Could you check a few things on this model? Use its own coordinates, in mm. Give positions to 0.01 mm unless a question says otherwise; leave off trailing zeros. Loops run counter-clockwise (first coordinate to the right, second up) from the corner with the lowest first, then second, coordinate; pieces in that order, holes last. Notation, with made-up numbers: (8.25, -11.75) -> (41.25, -11.75) arc R6 cw to (41.25, -0.75) -> close; hole circle Ø7 at (-26.5, 85). An arc over 180 degrees is marked (long way). Write item = value, one per line. Start each with the question number.
1) I want a section at C-C (z = 1.05). Count the separate pieces of the cut face and the enclosed holes in it, and give its area (3 significant figures).
2) I want a section at A-A (x = 160). List the corners of the cut face in (y, z) for me (3 decimals).
3) I'm going to push flat-ended pins straight in: pin 1 Ø1.5 at (x, y) = (117, 105) entering from -Z; pin 2 Ø1.6 at (y, z) = (13.5, 2) entering from +X; pin 3 Ø3 at (x, y) = (152.4, 106.807) entering from -Z. Where does each tip first touch, or does it pass through?
4) I need wall thicknesses on probe 1 along Y at (x, z) = (190.5, 2.55) (3 decimals); probe 2 along Y at (x, z) = (107.95, 1.85); probe 3 along X at (y, z) = (12.5, 2.7). Which ranges of each line are inside material? Lowest first, please. Write a range as from..to.
5) I want a section at B-B (y = 26). List the corners of the cut face in (x, z) for me (3 decimals).
6) If we mould it in two halves opening along Y, with no side actions, what happens to faces 1 (the face through (24.32, 56.86, 1.57)), 2 (the face through (36.573, 34.472, 1.61)), 3 (the face through (106, 82, 3.175))? For each: +Y half, -Y half, draft (parallel to the pull), parting line (faces both ways), or undercut.
Autodesk Inventor part; units mm, degrees
ref_plane "YZ Plane" through (0, 0, 0) normal (1, 0, 0) x (0, 1, 0)
ref_plane "XZ Plane" through (0, 0, 0) normal (0, 1, 0) x (-1, 0, 0)
ref_plane "XY Plane" through (0, 0, 0) normal (0, 0, 1) x (1, 0, 0)
sketch "Sketch1" plane through (0, 0, 0) normal (0, 0, 1) x (1, 0, 0)
  line L0 (0, 0) -> (215.9, 0)
  line L1 (215.9, 0) -> (215.9, 152.4)
  line L2 (215.9, 152.4) -> (0, 152.4)
  line L3 (0, 152.4) -> (0, 0)
  dimension "d0" = 215.9
  dimension "d1" = 152.4
extrude "Extrusion1" add sketch "Sketch1" along normal blind 3.175
sketch "Sketch2" plane through (0, 0, 3.175) normal (0, 0, 1) x (1, 0, 0)
  line L0 (215.9, 152.4) -> (0, 152.4) construction
  line L1 (107.95, 152.4) -> (107.95, 0) construction
  line L2 (0, 0) -> (215.9, 0)
  point P0 (25.273, 59.8875)
  point P1 (77.3049, 7.5)
  point P2 (190.627, 59.8875)
  point P3 (138.5951, 7.5)
  dimension "d5" = 30.6451
  dimension "d7" = 82.677
  dimension "d9" = 52.3875
  dimension "d10" = 7.5
hole "Hole1" at (25.273, 59.8875, 3.175) at (77.3049, 7.5, 3.175) at (190.627, 59.8875, 3.175) at (138.5951, 7.5, 3.175) direction (0, 0, -1) diameter 6.35 end through all
sketch "Sketch3" plane through (0, 0, 3.175) normal (0, 0, 1) x (1, 0, 0)
  line L0 (215.9, 152.4) -> (0, 152.4)
  line L1 (107.95, 152.4) -> (107.95, 0)
  line L2 (0, 0) -> (215.9, 0)
  line L3 (21.4376, 59.8875) -> (76.2, 7.5) construction
  line L4 (0, 152.4) -> (0, 0)
  line L5 (0, 130.175) -> (0, 78.2462)
  line L6 (3.175, 133.35) -> (107.95, 133.35)
  line L7 (0, 133.35) -> (0, 125.3708)
  line L8 (194.4624, 59.8875) -> (139.7, 7.5) construction
  line L9 (215.9, 152.4) -> (215.9, 78.2462)
  line L10 (215.9, 133.35) -> (215.9, 76.9596)
  line L11 (212.725, 133.35) -> (107.95, 133.35)
  line L12 (215.9, 130.175) -> (215.9, 125.3708)
  line L13 (75.9713, 0) -> (107.95, 0)
  line L14 (139.9287, 0) -> (107.95, 0)
  line L15 (215.9, 0) -> (215.9, 152.4)
  line L16 (107.95, 56.0437) -> (190.627, 56.0437) construction
  line L17 (0, 0) -> (215.9, 0)
  line L18 (143.7779, 0) -> (215.9, 69.9366)
  line L19 (72.1221, 0) -> (0, 69.9366)
  line L20 (0, 152.4) -> (0, 0)
  line L21 (72.1221, 0) -> (107.95, 0)
  line L22 (3.175, 133.35) -> (0, 133.35)
  line L23 (212.725, 133.35) -> (215.9, 133.35)
  point P0 (74.6275, 0)
  point P1 (0, 76.9596)
  point P2 (77.9849, 0)
  dimension "d20" = 19.05
  dimension "d36" = 135.881
  dimension "d37" = 135.881
  dimension "d41" = 35.8279
sketch "Sketch4" plane through (0, 0, 3.175) normal (0, 0, 1) x (1, 0, 0)
  arc A0 (80.4798, 20.1806) -> (74.13, 20.1806) centre (77.3049, 20.2) ccw
  circle A1 centre (77.3049, 7.5) radius 3.175
  circle A2 centre (77.3049, 7.5) radius 3.175
  line L0 (3.175, 133.35) -> (212.725, 133.35)
  line L1 (107.95, 133.35) -> (107.95, 0) construction
  line L2 (0, 0) -> (215.9, 0)
  arc A3 (141.77, 20.176) -> (135.4202, 20.176) centre (138.5951, 20.2) ccw
  arc A4 (74.1357, 7.5165) -> (80.474, 7.4806) centre (77.3049, 7.5) ccw
  circle A5 centre (138.5951, 7.5) radius 3.175
  arc A6 (135.4202, 7.5433) -> (141.77, 7.5433) centre (138.5951, 7.5) ccw
  line L3 (141.77, 20.176) -> (141.77, 7.476)
  circle A7 centre (138.5951, 7.5) radius 3.175
  line L4 (141.77, 20.176) -> (154.47, 20.176) construction
  line L5 (135.4202, 20.176) -> (135.4202, 7.476)
  line L6 (135.4202, 20.176) -> (148.1202, 20.176) construction
  line L7 (80.4798, 20.1806) -> (80.4798, 7.4806)
  line L8 (80.4798, 20.1806) -> (93.1798, 20.1806) construction
  line L9 (74.13, 20.1806) -> (74.1358, 7.4806)
  line L10 (74.13, 20.1806) -> (86.83, 20.1806) construction
  line L11 (74.13, 20.1806) -> (80.4798, 20.1806)
  line L12 (74.1358, 7.4806) -> (80.4798, 7.4806)
  line L13 (135.4202, 7.476) -> (141.77, 7.476)
  line L14 (135.4202, 20.176) -> (141.77, 20.176)
  line L15 (107.95, 0) -> (107.95, 152.4)
  line L16 (215.9, 152.4) -> (0, 152.4)
  line L17 (138.5951, 7.5) -> (107.95, 7.5)
  line L18 (138.5951, 20.2) -> (107.95, 20.2)
  line L19 (138.5951, 20.2) -> (169.2402, 20.2) construction
  point P0 (75.9713, 0)
  point P1 (139.9287, 0)
  point P2 (136.525, 7.4971)
  dimension "d29" = 6.35
  dimension "d30" = 12.7
  dimension "d44" = 90
  dimension "d45" = 90
  dimension "d46" = 90
  dimension "d48" = 12.7
  dimension "d49" = 12.7
  dimension "d50" = 12.7
  dimension "d117" = 180
extrude "Extrusion3" cut sketch "Sketch3" against normal blind 25.4 contours L9 L23 L11 L1 L0 | L1 L6 L22 L4 L0 | L2 L4 L19 | L18 L15 L2
extrude "Extrusion5" cut sketch "Sketch4" against normal blind 25.4 contours L11 A0 | L7 A1 L9 L11 | A1 L12 A4 L9 | L9 A4 L12 A1 | A4 L12 | L14 A3 | L3 A5 L5 L14 | A5 L13 | A5 L13
fillet "Fillet1" radius 3.175 6 edges at (0, 69.9366, 1.5875) (0, 133.35, 1.5875) (215.9, 133.35, 1.5875) (215.9, 69.9366, 1.5875) (143.7779, 0, 1.5875) (72.1221, 0, 1.5875)
sketch "Sketch5" plane through (0, 0, 3.175) normal (0, 0, 1) x (1, 0, 0)
  line L0 (73.4087, 0) -> (142.4913, 0)
  line L1 (73.4087, 0) -> (142.4913, 0)
  line L2 (107.95, 0) -> (107.95, 133.35)
  line L3 (212.725, 133.35) -> (3.175, 133.35)
  line L4 (107.95, 0) -> (241.3, 0) construction
  line L5 (107.95, 0) -> (107.95, 30.691)
  line L6 (122.6947, 0) -> (122.6947, 60.5028)
  line L7 (122.6947, 0) -> (183.1975, 0) construction
  circle A0 centre (107.95, 15.3455) radius 1.4986
  point P0 (0, 0)
  point P1 (93.2053, 60.5028)
  dimension "d56" = 90
  dimension "d58" = 90
  dimension "d59" = 60.5028
  dimension "d60" = 2.9972
  dimension "d61" = 14.7447
  dimension "d62" = 14.7447
  dimension "d63" = 60.5028
hole "Hole2" at (107.95, 15.3455, 3.175) at (93.2053, 60.5028, 3.175) at (122.6947, 60.5028, 3.175) at (107.95, 15.3455, 3.175) at (122.6947, 60.5028, 3.175) direction (0, 0, -1) diameter 2.9972 end through all
sketch "Sketch7" plane through (0, 0, 3.175) normal (0, 0, 1) x (1, 0, 0)
  line L0 (212.725, 133.35) -> (3.175, 133.35)
  line L1 (0, 130.175) -> (0, 71.2804)
  point P0 (0, 0)
  point P1 (19.05, 126.1872)
  point P2 (38.1, 106.807)
  point P3 (57.15, 126.1872)
  point P4 (76.2, 106.807)
  point P5 (95.25, 126.1872)
  point P6 (114.3, 106.807)
  point P7 (133.35, 126.1872)
  point P8 (152.4, 106.807)
  point P9 (171.45, 126.1872)
  point P10 (190.5, 106.807)
  dimension "d83" = 7.1628
  dimension "d84" = 19.05
  dimension "d85" = 7.1628
  dimension "d89" = 26.543
  dimension "d90" = 26.543
  dimension "d94" = 38.1
  dimension "d95" = 57.15
  dimension "d96" = 76.2
  dimension "d97" = 7.1628
  dimension "d98" = 95.25
  dimension "d99" = 26.543
  dimension "d100" = 114.3
  dimension "d102" = 7.1628
  dimension "d103" = 133.35
  dimension "d104" = 26.543
  dimension "d105" = 152.4
  dimension "d106" = 7.1628
  dimension "d107" = 171.45
  dimension "d108" = 26.543
  dimension "d109" = 190.5
hole "Hole4" at (19.05, 126.1872, 3.175) at (38.1, 106.807, 3.175) at (57.15, 126.1872, 3.175) at (76.2, 106.807, 3.175) at (95.25, 126.1872, 3.175) at (114.3, 106.807, 3.175) at (133.35, 126.1872, 3.175) at (152.4, 106.807, 3.175) at (171.45, 126.1872, 3.175) at (190.5, 106.807, 3.175) direction (0, 0, -1) diameter 3.556 end through all
equation "\"d37\" = d36"
equation "\"d48\" = d30"
equation "\"d49\" = d50"
properties part number "new pulley plate"
Answer list:
q1.separate_pieces = 1
q1.enclosed_holes = 17
q1.area = 23,300 mm^2
q2.outline = (15.731, 0) -> (133.35, 0) -> (133.35, 3.175) -> (15.731, 3.175) -> close
q3.pin_1 = 0
q3.pin_2 = 158.52
q3.pin_3 = through
q4.probe_1 = 45.306..56.715, 63.06..105.029, 108.585..133.35
q4.probe_2 = 0..13.85, 16.84..133.35
q4.probe_3 = 59.23..74.13, 80.48..135.42, 141.77..156.67
q5.outline = (45.31, 0) -> (170.59, 0) -> (170.59, 3.175) -> (45.31, 3.175) -> close
q6.face_1 = undercut
q6.face_2 = -Y half
q6.face_3 = draft
